from build123d import *

# Parameters (mm, degrees)
F0_W     = 266.7
F0_H     = 152.4
F0_R     = 19.05
F1_DEPTH = 50.8
F2_R     = 6.35


with BuildPart() as f1:
    # F0 (on Front) → F1 (new body)
    with BuildSketch(Plane.XZ):
        with Locations((1.909529, 0)):
            Rectangle(F0_W, F0_H)
        with Locations((-82.55, 0)):
            Circle(F0_R, mode=Mode.SUBTRACT)
        with BuildLine():
            ThreePointArc((-19.05, 0), (0, 19.05), (19.05, 0))
            ThreePointArc((19.05, 0), (0, -19.05), (-19.05, 0))
        make_face(mode=Mode.SUBTRACT)
        with BuildLine():
            ThreePointArc((103.550499, 0), (84.500499, -19.05), (65.450499, 0))
            ThreePointArc((65.450499, 0), (84.500499, 19.05), (103.550499, 0))
        make_face(mode=Mode.SUBTRACT)
    extrude(amount=F1_DEPTH)

    # F2
    f2_edges = [f1.edges().sort_by_distance(p)[0] for p in [
        (1.909529, -50.8, -76.2),
        (-131.440471, -25.4, -76.2),
        (135.259529, -25.4, -76.2),
        (1.909529, 0, -76.2),
        (-131.440471, 0, 0),
        (135.259529, -25.4, 76.2),
        (-131.440471, -25.4, 76.2),
        (1.909529, 0, 76.2),
        (1.909529, -50.8, 76.2),
        (135.259529, 0, 0),
        (135.259529, -50.8, 0),
    ]]
    fillet(f2_edges, radius=F2_R)


solid = f1.part
Input: part model. Units: mm. Frame: model coordinates. Give positions to 0.01 mm unless a question says otherwise; leave off trailing zeros. Order: outer loops, then holes, each group sorted by start corner. A loop starts at its lowest first (then second) coordinate and runs counter-clockwise, first axis right, second up.
Q1. Section C-C on y = -25. Output: boundary loops of the cut face in (x, z), and give its area (3 significant figures).
Checked values:
outline: (-131.44, -69.85) arc R6.35 ccw to (-125.09, -76.2) - (128.91, -76.2) arc R6.35 ccw to (135.26, -69.85) - (135.26, 69.85) arc R6.35 ccw to (128.91, 76.2) - (-125.09, 76.2) arc R6.35 ccw to (-131.44, 69.85) - close; hole circle Ø38.1 at (-82.55, 0); hole circle Ø38.1 at (0, 0); hole circle Ø38.1 at (84.5, 0)
area: 37,200 mm2
Q2. Section B-B on x = -82.55. Output: boundary loops of the cut face in (y, z), and give its area (3 significant figures).
Checked values:
outline: (-50.8, -69.85) arc R6.35 ccw to (-44.45, -76.2) - (-6.35, -76.2) arc R6.35 ccw to (0, -69.85) - (0, -19.05) - (-50.8, -19.05) - close; (-50.8, 19.05) - (0, 19.05) - (0, 69.85) arc R6.35 ccw to (-6.35, 76.2) - (-44.45, 76.2) arc R6.35 ccw to (-50.8, 69.85) - close
area: 5,770 mm2
Q3. Section A-A on z = 0. Output: boundary loops of the cut face in (x, y).
Checked values:
outline: (-131.44, -50.8) - (-101.6, -50.8) - (-101.6, 0) - (-125.09, 0) arc R6.35 ccw to (-131.44, -6.35) - close; (-63.5, -50.8) - (-19.05, -50.8) - (-19.05, 0) - (-63.5, 0) - close; (19.05, -50.8) - (65.45, -50.8) - (65.45, 0) - (19.05, 0) - close; (103.55, -50.8) - (128.91, -50.8) arc R6.35 ccw to (135.26, -44.45) - (135.26, -6.35) arc R6.35 ccw to (128.91, 0) - (103.55, 0) - close
Q4. Section D-D on x = 2. Output: boundary loops of the cut face in (y, z), and give its area (3 significant figures).
Checked values:
outline: (-50.8, -69.85) arc R6.35 ccw to (-44.45, -76.2) - (-6.35, -76.2) arc R6.35 ccw to (0, -69.85) - (0, -18.94) - (-50.8, -18.94) - close; (-50.8, 18.94) - (0, 18.94) - (0, 69.85) arc R6.35 ccw to (-6.35, 76.2) - (-44.45, 76.2) arc R6.35 ccw to (-50.8, 69.85) - close
area: 5,780 mm2
Q5. Ray query, probe 1 along Z at (x, y) = (-81.5, -42); probe 2 along X at (y, z) = (-40.5, 4); probe 3 along X at (y, z) = (-25.5, 6). Return the intervals inside material, ascending.
Checked values:
probe 1: z = -76.2 to -19.02, 19.02 to 76.2
probe 2: x = -131.44 to -101.18, -63.92 to -18.63, 18.63 to 65.88, 103.13 to 135.26
probe 3: x = -131.44 to -100.63, -64.47 to -18.08, 18.08 to 66.42, 102.58 to 135.26
Q6. Draft query along Z for faces 1 (the cylindrical face through (-15.12, -25.04, 11.59)), 2 (the cylindrical face through (3.69, -1.91, -74.39)), 3 (the cylindrical face through (133.45, -48.89, 0.98)), 4 (the flat face through (0, -25, 76.2)). Return one class per face: +Z half, -Z half, draft (parallel to the pull), parting line (faces both ways), or undercut.
Checked values:
face 1: undercut
face 2: -Z half
face 3: draft
face 4: +Z half
